```python
from build123d import *

# Parameters (mm, degrees)
SKETCH1_W           = 15
SKETCH1_H           = 11.5
BOSS_EXTRUDE1_DEPTH = 1.5
SKETCH4_W           = 1.5
SKETCH4_H           = 11.5
BOSS_EXTRUDE2_DEPTH = 10
BOSS_EXTRUDE3_DEPTH = 3.5
CUT_EXTRUDE1_DEPTH  = 1.5
SKETCH12_R          = 1.5
CUT_EXTRUDE3_DEPTH  = 19.366069258
FILLET1_R           = 2
FILLET2_R           = 0.5


with BuildPart() as part:
    # Sketch1 → Boss-Extrude1 (new body)
    with BuildSketch(Plane(origin=(0, 0, 0), x_dir=(1, 0, 0), z_dir=(0, 1, 0))):
        Rectangle(SKETCH1_W, SKETCH1_H)
    extrude(amount=BOSS_EXTRUDE1_DEPTH)

    # Sketch4 → Boss-Extrude2 (add)
    with BuildSketch(Plane.XZ):
        with Locations((-6.75, 0)):
            Rectangle(SKETCH4_W, SKETCH4_H)
        with Locations((6.75, 0)):
            Rectangle(SKETCH4_W, SKETCH4_H)
    extrude(amount=BOSS_EXTRUDE2_DEPTH)

    # Sketch5 → Boss-Extrude3 (add)
    with BuildSketch(Plane.XZ.offset(10)):
        with BuildLine():
            Line((-6, -5.75), (-11.5, -5.75))
            ThreePointArc((-11.5, -5.75), (-15.5, -1.75), (-11.5, 2.25))
            Line((-11.5, 2.25), (-6, 2.25))
            Line((-6, 2.25), (-6, -5.75))
        make_face()
        with BuildLine():
            Line((6, -5.75), (11.5, -5.75))
            ThreePointArc((11.5, -5.75), (15.5, -1.75), (11.5, 2.25))
            Line((11.5, 2.25), (6, 2.25))
            Line((6, 2.25), (6, -5.75))
        make_face()
    extrude(amount=-BOSS_EXTRUDE3_DEPTH)

    # Sketch10 → Cut-Extrude1 (cut)
    with BuildSketch(Plane(origin=(0, -6.5, 0), x_dir=(1, 0, 0), z_dir=(0, 1, 0))):
        Polygon((-8.5, 3.482050808), (-11.5, 5.214101615), (-14.5, 3.482050808), (-14.5, 0.017949192), (-11.5, -1.714101615), (-8.5, 0.017949192), align=None)
    cut_extrude1 = extrude(amount=-CUT_EXTRUDE1_DEPTH, mode=Mode.SUBTRACT)

    # Sketch12 → Cut-Extrude3 (cut, through all)
    with BuildSketch(Plane(origin=(0, -6.5, 0), x_dir=(1, 0, 0), z_dir=(0, 1, 0))):
        with Locations(Location((-11.5, 1.75, 0), (0, 0, 270))):
            Circle(SKETCH12_R)
    cut_extrude3 = extrude(amount=-CUT_EXTRUDE3_DEPTH, mode=Mode.SUBTRACT)

    # Mirror1: Cut-Extrude1, Cut-Extrude3 across plane
    add(cut_extrude1.mirror(Plane(origin=(0, 0, 0), x_dir=(0, 0, 1), z_dir=(1, 0, 0))), mode=Mode.SUBTRACT)
    add(cut_extrude3.mirror(Plane(origin=(0, 0, 0), x_dir=(0, 0, 1), z_dir=(1, 0, 0))), mode=Mode.SUBTRACT)

    # Fillet1
    fillet1_edges = [part.edges().sort_by_distance(p)[0] for p in [
        (7.5, 1.5, 0),
        (-7.5, 1.5, 0),
    ]]
    fillet(fillet1_edges, radius=FILLET1_R)

    # Fillet2
    fillet2_edges = [part.edges().sort_by_distance(p)[0] for p in [
        (-6, 0, 0),
        (6, 0, 0),
        (-7.5, -6.5, -1.75),
        (-7.5, -8.25, 2.25),
        (7.5, -8.25, 2.25),
        (7.5, -6.5, -1.75),
    ]]
    fillet(fillet2_edges, radius=FILLET2_R)


solid = part.part
```
Check sheet for the modelled part. Datum: model origin and axes. Units: mm. A direction names the side the tool comes from. Give positions to 0.01 mm unless a question says otherwise; leave off trailing zeros. Loops run counter-clockwise (first coordinate to the right, second up) from the corner with the lowest first, then second, coordinate; pieces in that order, holes last. Notation, with made-up numbers: (-12, 73) - (34, 73) arc R18 ccw to (34, 88) - close; hole circle Ø2 at (48.5, 54.5). An arc over 180 degrees is marked (long way). One line per question, with ' | ' between items. Start each with the question number.
1. Gauge pin test, flat ends, axial feed: pin 1 Ø4 at (x, y) = (10.5, -9) entering from +Z; pin 2 Ø3 at (x, z) = (-10.5, -2) entering from +Y; pin 3 Ø3 at (y, z) = (-9, 1) entering from +X. Record the tip position at first contact, or that the pin passes through.
2. Draft check along Z on faces 1 (the cylindrical face through (15.5, -8.3, -1.8)), 2 (the flat face through (0, 0, 0)), 3 (the flat face through (-13, -8, -1)), 4 (the flat face through (-14.5, -7, -2)). Enter one of: released by +Z, released by -Z, zero draft, split by the parting line, or undercut.
3. Set-up check for faces 5 (the flat face through (7.5, -4, 1)), 6 (the flat face through (-8.5, -7, -2)), 7 (the flat face through (-7.5, -4, 1)): record each of +Z, -Z, +X, -X, +Y, -Y from which the full face is reachable in a straight line by a thin tool's end or side.
4. Cross-section at C-C, the plane z = -1.75. Give the number of separate pieces and of enclosed holes in the cut face, plus the area to 3 significant figures.
5. Cross-section at D-D, the plane x = 11. Enter the section's corners in (y, z), plus the area to 3 significant figures.
6. Material ranges on line 1 along X through (y, z) = (-8.7, -1.75); line 2 along X through (y, z) = (-1.5, -2.25); line 3 along X through (y, z) = (-8.25, 1.25), recorded low to high. Write a range as [from, to].
7. Cross-section at A-A, the plane y = -9. Enter the section's corners in (x, z), plus the area to 3 significant figures.
8. Cross-section at B-B, the plane y = -4.25. Enter the section's corners in (x, z), plus the area to 3 significant figures.
Check result:
1) pin 1: stops at z = 2.25 | pin 2: stops at y = -8 | pin 3: stops at x = 15.3
2) face 1: split by the parting line | face 2: zero draft | face 3: undercut | face 4: undercut
3) face 5: +Z, +X, +Y | face 6: +Y | face 7: +Z, -X, +Y
4) separate pieces: 3 | enclosed holes: 0 | area: 77.0 mm2
5) outline: (-10, -5.75) - (-6.5, -5.75) - (-6.5, -4.93) - (-8, -4.93) - (-8, -3.16) - (-10, -3.16) - close; (-10, -0.34) - (-8, -0.34) - (-8, 1.43) - (-6.5, 1.43) - (-6.5, 2.25) - (-10, 2.25) - close | area: 12.8 mm2
6) line 1: x = [-15.5, -13], [-10, -6], [6, 10], [13, 15.5] | line 2: x = [-7.5, -6], [6, 7.5] | line 3: x = [-14.15, -6], [6, 14.15]
7) outline: (-11.5, -5.75) - (-6, -5.75) - (-6, 5.75) - (-7.5, 5.75) - (-7.5, 2.75) arc R0.5 cw to (-8, 2.25) - (-11.5, 2.25) arc R4 ccw to start; (6, -5.75) - (11.5, -5.75) arc R4 ccw to (11.5, 2.25) - (8, 2.25) arc R0.5 cw to (7.5, 2.75) - (7.5, 5.75) - (6, 5.75) - close; hole circle Ø3 at (-11.5, -1.75); hole circle Ø3 at (11.5, -1.75) | area: 135 mm2
8) outline: (-7.5, -5.75) - (-6, -5.75) - (-6, 5.75) - (-7.5, 5.75) - close; (6, -5.75) - (7.5, -5.75) - (7.5, 5.75) - (6, 5.75) - close | area: 34.5 mm2
